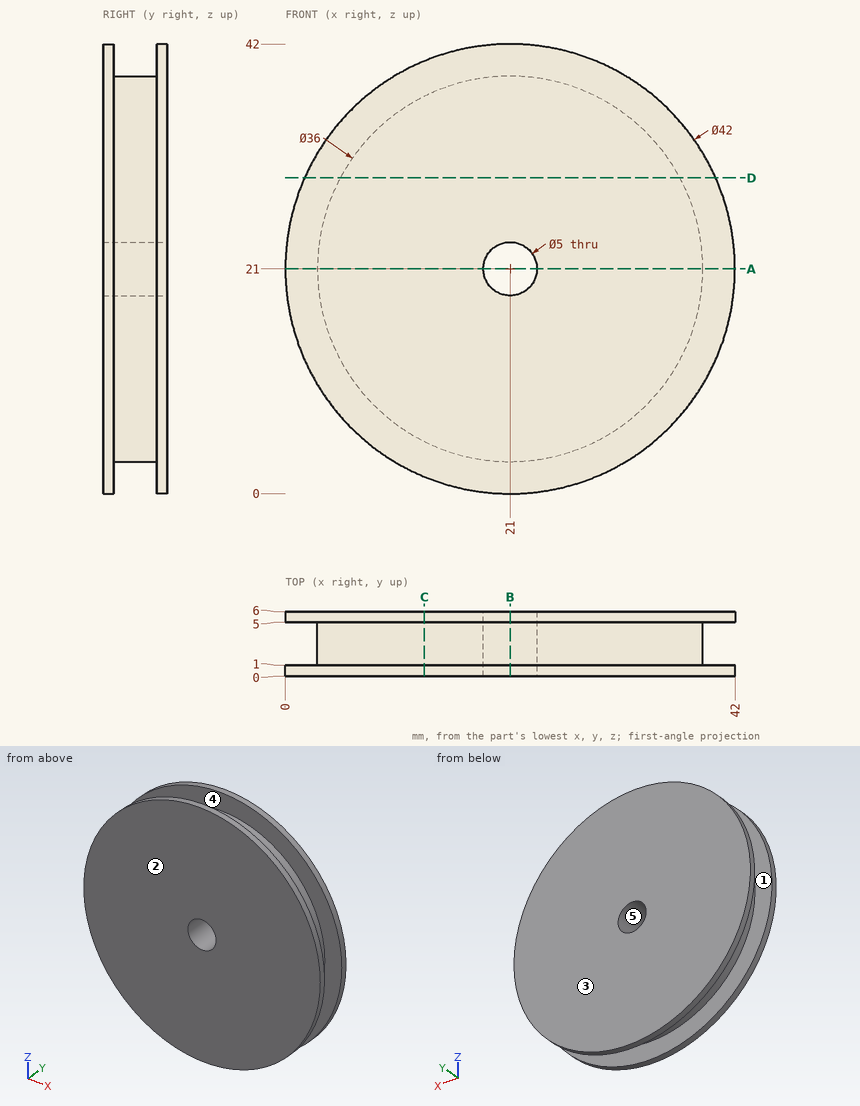
The drawing under review shows one solid part. Ordinate dimensions are in mm from its lowest x, y, z. A direction names the side the tool comes from. Round coordinates to 2 decimals unless told otherwise and drop trailing zeros. Order: outer loops, then holes, each group sorted by start corner. A loop starts at its lowest first (then second) coordinate and runs counter-clockwise, first axis right, second up. Notation, with made-up numbers: M 65,-30 L 70,-30 A17 ccw 70,-26 Z; hole C 81,-14.5 d8. An arc over 180 degrees is marked long. Answer as CSV lines item,"result". Start each with the question number.
1) Add section C-C (x = 13). Give the boundary of the cut face in (y, z).
2) Add section D-D (z = 29.5). Give the boundary of the cut face in (x, y).
3) Add section A-A (z = 21). Give the boundary of the cut face in (x, y), then the cut area to 3 significant figures.
4) For pin 1 Ø1 at (y, z) = (2.5, 18) entering from -X; pin 2 Ø4.5 at (x, z) = (21, 21) entering from +Y, all flat-tipped, find the tip position at first contact; note any pin that passes through.
5) The part is to be moulded in two halves that separate along Y. For the marked faces 3, 4 and 5, say which applies: +Y half, -Y half, draft (parallel to the pull), parting line (faces both ways), or undercut.
6) Tool access review of the marked faces 1 and 2: name each direction out of +Z, -Z, +X, -X, +Y, -Y from which nothing blocks a thin tool from reaching the whole face with its end or side.
7) Wall thickness on line 1 along Y through (x, z) = (40.5, 26.5); line 2 along Z through (x, y) = (21, 4); line 3 along Z through (x, y) = (32, 2.9): over which ranges is each line inside the solid? List them lowest first. Write a range as [from, to].
8) Add section B-B (x = 21). Give the boundary of the cut face in (y, z).
Resolved:
1,outline,"M 0,1.58 L 1,1.58 L 1,4.88 L 5,4.88 L 5,1.58 L 6,1.58 L 6,40.42 L 5,40.42 L 5,37.12 L 1,37.12 L 1,40.42 L 0,40.42 Z"
2,outline,"M 1.8,0 L 40.2,0 L 40.2,1 L 36.87,1 L 36.87,5 L 40.2,5 L 40.2,6 L 1.8,6 L 1.8,5 L 5.13,5 L 5.13,1 L 1.8,1 Z"
3,outline,"M 0,0 L 18.5,0 L 18.5,6 L 0,6 L 0,5 L 3,5 L 3,1 L 0,1 Z; M 23.5,0 L 42,0 L 42,1 L 39,1 L 39,5 L 42,5 L 42,6 L 23.5,6 Z"
3,area,"198 mm^2"
4,pin 1,"x = 3.17"
4,pin 2,"through"
5,face 3,"+Y half"
5,face 4,"undercut"
5,face 5,"draft"
6,face 1,"none"
6,face 2,"+Z, -Z, +X, -X, -Y"
7,line 1,"[0, 1], [5, 6]"
7,line 2,"[3, 18.5], [23.5, 39]"
7,line 3,"[6.75, 35.25]"
8,outline,"M 0,0 L 1,0 L 1,3 L 5,3 L 5,0 L 6,0 L 6,18.5 L 0,18.5 Z; M 0,23.5 L 6,23.5 L 6,42 L 5,42 L 5,39 L 1,39 L 1,42 L 0,42 Z"
